Here's how the part is built. I have some questions about the finished solid (model axes, mm). A direction names the side the tool comes from. Coordinates: 2 decimals unless noted, no trailing zeros. Write each loop counter-clockwise with the first axis right and the second up, starting at its lowest first coordinate (ties: lowest second). Pieces come first, ordered by that corner, then holes.
```python
from build123d import *

# Parameters (mm, degrees)
ESQUISSE1_W                  = 34
ESQUISSE1_H                  = 28
BOSS_EXTRU_1_DEPTH           = 9
ESQUISSE2_W                  = 20
ESQUISSE2_H                  = 9
BOSS_EXTRU_2_DEPTH           = 9
ENL_V_MAT_EXTRU_1_DEPTH      = 52.048996072
ENL_V_MAT_EXTRU_1_DEPTH_BACK = 52.048996072
ENL_V_MAT_EXTRU_2_DEPTH      = 52.048996072
ENL_V_MAT_EXTRU_2_DEPTH_BACK = 52.048996072
ESQUISSE4_R                  = 1.65


with BuildPart() as part:
    # Esquisse1 → Boss.-Extru.1 (new body)
    with BuildSketch(Plane.XY):
        with Locations((17, 14)):
            Rectangle(ESQUISSE1_W, ESQUISSE1_H)
    extrude(amount=BOSS_EXTRU_1_DEPTH)

    # Esquisse2 → Boss.-Extru.2 (add)
    with BuildSketch(Plane.XY.offset(9)):
        with Locations((17, 32.5)):
            Rectangle(ESQUISSE2_W, ESQUISSE2_H)
    extrude(amount=-BOSS_EXTRU_2_DEPTH)

    # Esquisse3 → Enlèv. mat.-Extru.1 (cut, two sides: drawn at the far end of the back side and taken through both)
    with BuildSketch(Plane.XY.offset(9).offset(-ENL_V_MAT_EXTRU_1_DEPTH_BACK)):
        with BuildLine():
            Line((4.525126266, 28), (7, 30.474873734))
            ThreePointArc((7, 30.474873734), (7.070710678, 27.929289322), (4.525126266, 28))
        make_face()
        with BuildLine():
            Line((29.474873734, 28), (27, 30.474873734))
            ThreePointArc((27, 30.474873734), (26.929289322, 27.929289322), (29.474873734, 28))
        make_face()
    extrude(amount=ENL_V_MAT_EXTRU_1_DEPTH + ENL_V_MAT_EXTRU_1_DEPTH_BACK, mode=Mode.SUBTRACT)

    # Esquisse4 → Enlèv. mat.-Extru.2 (cut, two sides: drawn at the far end of the back side and taken through both)
    with BuildSketch(Plane.XY.offset(9).offset(-ENL_V_MAT_EXTRU_2_DEPTH_BACK)):
        with Locations((7, 24)):
            Circle(ESQUISSE4_R)
        with Locations(Location((27, 24, 0), (0, 0, 180))):
            Circle(ESQUISSE4_R)
        with Locations((27, 4)):
            Circle(ESQUISSE4_R)
        with Locations(Location((7, 4, 0), (0, 0, 180))):
            Circle(ESQUISSE4_R)
    extrude(amount=ENL_V_MAT_EXTRU_2_DEPTH + ENL_V_MAT_EXTRU_2_DEPTH_BACK, mode=Mode.SUBTRACT)


solid = part.part
```
1) Imagine slicing it at A-A on z = 3.5. Please give me the cut outline in (x, y), then the cut area to 3 significant figures.
Values follow:
outline: (0, 0) - (34, 0) - (34, 28) - (29.47, 28) arc R1.75 cw (long way) to (27, 30.47) - (27, 37) - (7, 37) - (7, 30.47) arc R1.75 cw (long way) to (4.53, 28) - (0, 28) - close; hole circle Ø3.3 at (7, 4); hole circle Ø3.3 at (7, 24); hole circle Ø3.3 at (27, 4); hole circle Ø3.3 at (27, 24)
area: 1,090 mm2
2) On a 3-axis mill with a long thin cutter (end or side, diameter ignored), from which of +Z, -Z, +X, -X, +Y, -Y can I reach the whole of each face in a straight line? I mean faces 1 (the face through (27, 34, 5)), 2 (the face through (8.65, 3.93, 4.44)), 3 (the face through (2, 28, 4)). Say none if no direction works.
Values follow:
face 1: +Z, -Z, +X, +Y
face 2: +Z, -Z
face 3: +Z, -Z, -X, +Y
3) Will these pins go through, and if not, where does the flat tip stop? pin 1 (3.5 mm diameter, centred on y = 33.5, z = 4.5, fed in from -X); pin 2 (1.5 mm diameter, centred on x = 6.5, y = 23.5, fed in from -Z); pin 3 (5 mm diameter, centred on x = 2.5, z = 2.5, fed in from +Y); pin 4 (2 mm diameter, centred on y = 33.5, z = 6, fed in from +X).
Values follow:
pin 1: stops at x = 7
pin 2: passes through
pin 3: stops at y = 28
pin 4: stops at x = 27
4) Imagine slicing it at C-C on x = 28. Please give me the cut outline in (y, z).
Values follow:
outline: (0, 0) - (2.69, 0) - (2.69, 9) - (0, 9) - close; (5.31, 0) - (22.69, 0) - (22.69, 9) - (5.31, 9) - close; (25.31, 0) - (27.42, 0) - (27.42, 9) - (25.31, 9) - close
5) We'd pull the mould along Y, two halves only. Please class faces 4 (the face through (32, 28, 4)), 5 (the face through (25.35, 4.07, 4.44)), 6 (the face through (34, 14, 4)): pulls with the +Y half, pulls with the -Y half, needs draft (parallel to the pull), parting line crosses it, or undercut.
Values follow:
face 4: pulls with the +Y half
face 5: undercut
face 6: needs draft
6) Imagine slicing it at D-D on y = 34. Please give me the cut outline in (x, z).
Values follow:
outline: (7, 0) - (27, 0) - (27, 9) - (7, 9) - close
7) Imagine slicing it at B-B on y = 24. Please give me the cut outline in (x, z), then the cut area to 3 significant figures.
Values follow:
outline: (0, 0) - (5.35, 0) - (5.35, 9) - (0, 9) - close; (8.65, 0) - (25.35, 0) - (25.35, 9) - (8.65, 9) - close; (28.65, 0) - (34, 0) - (34, 9) - (28.65, 9) - close
area: 247 mm2
8) I need wall thicknesses on probe 1 along X at (y, z) = (23, 5); probe 2 along X at (y, z) = (23.5, 4.75); probe 3 along Y at (x, z) = (6.5, 6). Which ranges of each line are inside material? Lowest first, please.
Values follow:
probe 1: x = 0 to 5.69, 8.31 to 25.69, 28.31 to 34
probe 2: x = 0 to 5.43, 8.57 to 25.43, 28.57 to 34
probe 3: y = 0 to 2.43, 5.57 to 22.43, 25.57 to 27.55
